from build123d import *

# Parameters (mm, degrees)
SKETCH1_W           = 25.4
SKETCH1_H           = 27.94
SKETCH1_W_2         = 21.59
SKETCH1_H_2         = 24.13
BOSS_EXTRUDE1_DEPTH = 3.175
FILLET1_R           = 0.635


with BuildPart() as part:
    # Sketch1 → Boss-Extrude1 (new body)
    with BuildSketch(Plane.XY):
        Rectangle(SKETCH1_W, SKETCH1_H)
        Rectangle(SKETCH1_W_2, SKETCH1_H_2, mode=Mode.SUBTRACT)
    extrude(amount=BOSS_EXTRUDE1_DEPTH)

    # Fillet1
    fillet1_edges = [part.edges().sort_by_distance(p)[0] for p in [
        (10.795, 0, 0),
        (0, 12.065, 0),
        (-10.795, 0, 0),
        (0, -12.065, 0),
        (10.795, 0, 3.175),
        (0, 12.065, 3.175),
        (-10.795, 0, 3.175),
        (0, -12.065, 3.175),
        (12.7, -13.97, 1.5875),
        (-12.7, -13.97, 1.5875),
        (-12.7, 13.97, 1.5875),
        (12.7, 13.97, 1.5875),
    ]]
    fillet(fillet1_edges, radius=FILLET1_R)


solid = part.part
CAD build for the part. Positions are in the model's coordinates, mm. A direction names the side the tool comes from. Round coordinates to 2 decimals unless told otherwise and drop trailing zeros. Order: outer loops, then holes, each group sorted by start corner. A loop starts at its lowest first (then second) coordinate and runs counter-clockwise, first axis right, second up. Notation, with made-up numbers: (-20, -29.75) -> (18, -29.75) arc R27 ccw to (18, -6.75) -> close; hole circle Ø9 at (-38.5, 31). An arc over 180 degrees is marked (long way). Write each question's results on one line, items separated by ' | '.
1. 3-axis set-ups, long thin cutter, end or side, ignore diameter. For faces 5 (the face through (0, 12.065, 2)), 6 (the face through (0, -13.97, 2)): which of +Z, -Z, +X, -X, +Y, -Y reach the whole face in a straight line?
Findings below:
face 5: +Z, -Z | face 6: +Z, -Z, +X, -X, -Y
2. Cut at A-A (y = 8.75). Give the cut face in (x, z) (3 decimals).
Findings below:
outline: (-12.7, 0) -> (-11.43, 0) arc R0.635 ccw to (-10.795, 0.635) -> (-10.795, 2.54) arc R0.635 ccw to (-11.43, 3.175) -> (-12.7, 3.175) -> close; (10.795, 0.635) arc R0.635 ccw to (11.43, 0) -> (12.7, 0) -> (12.7, 3.175) -> (11.43, 3.175) arc R0.635 ccw to (10.795, 2.54) -> close
3. Cut at B-B (x = -0.75). Give the cut face in (y, z) (3 decimals), plus the area to 3 significant figures.
Findings below:
outline: (-13.97, 0) -> (-12.7, 0) arc R0.635 ccw to (-12.065, 0.635) -> (-12.065, 2.54) arc R0.635 ccw to (-12.7, 3.175) -> (-13.97, 3.175) -> close; (12.065, 0.635) arc R0.635 ccw to (12.7, 0) -> (13.97, 0) -> (13.97, 3.175) -> (12.7, 3.175) arc R0.635 ccw to (12.065, 2.54) -> close | area: 11.8 mm²
4. Flat gauge pin, fed straight in: P1, Ø6, axis at x = 3, y = 8, coming from the -Z side. Where does the tip first touch, or does it go through?
Findings below:
P1: passes through
5. Pull direction X, two halves, no side cores. Call faces 1 (the face through (12.7, 0, 2)), 2 (the face through (-12, 0, 0)), 3 (the face through (-12.7, 0, 2)), 4 (the face through (10.795, 0, 2)): pulls with the +X half, pulls with the -X half, needs draft (parallel to the pull), parting line crosses it, or undercut.
Findings below:
face 1: pulls with the +X half | face 2: needs draft | face 3: pulls with the -X half | face 4: undercut
6. Wall check: line 1 along X through (y, z) = (-12, 1.05) (3 decimals); line 2 along Y through (x, z) = (-5.5, 1.3) (3 decimals); line 3 along X through (y, z) = (-10.5, 3). Give the ranges that are in metal, low to high. Write a range as [from, to].
Findings below:
line 1: x = [-12.7, -10.795], [10.795, 12.7] | line 2: y = [-13.97, -12.065], [12.065, 13.97] | line 3: x = [-12.7, -10.99], [10.99, 12.7]
